```python
from build123d import *

# Parameters (mm, degrees)
SKETCH_W             = 18
SKETCH_H             = 18
PAD_DEPTH            = 8
POCKET_DEPTH         = 18.001
POCKET001_DEPTH      = 9.001
POCKET001_DEPTH_BACK = 9.001
FILLET_R             = 2
THICKNESS_T          = -1


with BuildPart() as part:
    # Sketch → Pad (new body)
    with BuildSketch(Plane.XY):
        Rectangle(SKETCH_W, SKETCH_H)
    extrude(amount=PAD_DEPTH)

    # Sketch001 (on Face1 of Pad) → Pocket (cut, through all)
    with BuildSketch(Plane.XZ.offset(9)):
        Polygon((-9, 8), (-9, 0), (-7, 8), align=None)
        Polygon((9, 8), (9, 0), (7, 8), align=None)
    extrude(amount=-POCKET_DEPTH, mode=Mode.SUBTRACT)

    # Sketch002 → Pocket001 (cut, two sides)
    with BuildSketch(Plane.YZ) as pocket001_sk:
        Polygon((-9, 8), (-7, 8), (-9, 0), align=None)
        Polygon((9, 8), (7, 8), (9, 0), align=None)
    extrude(amount=-POCKET001_DEPTH, mode=Mode.SUBTRACT)
    extrude(pocket001_sk.sketch, amount=POCKET001_DEPTH_BACK, mode=Mode.SUBTRACT)

    # Fillet
    fillet_edges = [part.edges().sort_by_distance(p)[0] for p in [
        (-8, 8, 4),
        (-8, -8, 4),
        (8, -8, 4),
        (8, 8, 4),
    ]]
    fillet(fillet_edges, radius=FILLET_R)

    # Thickness
    thickness_openings = [part.faces().sort_by_distance(p)[0] for p in [
        (0, 0, 0),
    ]]
    offset(amount=THICKNESS_T, openings=thickness_openings, kind=Kind.INTERSECTION)


solid = part.part
```
Verification items for the finished model (mm, model axes). A direction names the side the tool comes from. Coordinates: 2 decimals unless noted, no trailing zeros. Write each loop counter-clockwise with the first axis right and the second up, starting at its lowest first coordinate (ties: lowest second). Pieces come first, ordered by that corner, then holes. Notation, with made-up numbers: M 46,79.5 L 87,79.5 A13 cw 87,103.5 Z; hole C 35,86.5 d10. An arc over 180 degrees is marked long. Answer as a JSON object with one key per item and string values. Group by question number.
(1) Release check for a two-part mould opening along X. For faces 3 (the face through (6.8, -6.78, 3.59)), 4 (the face through (-8, 0, 4)), 5 (the face through (0, 8, 4)) record: +X half, -X half, draft (parallel to the pull), parting line (faces both ways), or undercut.
(2) Tool access check on faces 1 (the face through (0, 0, 8)), 2 (the face through (0.1, -7.08, 3.55)). Record the directions out of +Z, -Z, +X, -X, +Y, -Y that give a thin tool (end or side, any length) a straight path to the whole face; none if there is none.
(3) Material ranges on line 1 (X direction, y = -6.5, z = 5.5); line 2 (X direction, y = -0.75, z = 5.75); line 3 (Y direction, x = 0.5, z = 1.5) (3 decimals), recorded low to high.
(4) Cross-section at A-A, the plane y = -3. Record the cut outline in (x, z).
(5) Gauge pin test, flat ends, axial feed: pin 1 (1.5 mm diameter, centred on y = -6.5, z = 2, fed in from -X); pin 2 (4 mm diameter, centred on x = -2.5, z = 5, fed in from -Y); pin 3 (6 mm diameter, centred on x = 2.5, y = -0.5, fed in from -Z). Record the tip position at first contact, or that the pin passes through.
Reply:
{
 "1": {"face 3": "undercut", "face 4": "-X half", "face 5": "draft"},
 "2": {"face 1": "+Z, +X, -X, +Y, -Y", "face 2": "-Z"},
 "3": {"line 1": "-7.45 to -6.05, 6.05 to 7.45", "line 2": "-7.56 to -6.53, 6.53 to 7.56", "line 3": "-8.625 to -7.594, 7.594 to 8.625"},
 "4": {"outline": "M -9,0 L -7.97,0 L -6.22,7 L 6.22,7 L 7.97,0 L 9,0 L 7,8 L -7,8 Z"},
 "5": {"pin 1": "x = -8.69", "pin 2": "y = -8.25", "pin 3": "z = 7"}
}
